from build123d import *

# Parameters (mm, degrees)
P_IDAT_VYSUNUT_M1_DEPTH  = 20
P_IDAT_VYSUNUT_M2_DEPTH  = 10
P_IDAT_START             = -16
P_IDAT_VYSUNUT_M3_DEPTH  = 12
ODEBRAT_START            = -4
SKICA4_R                 = 4.1
ODEBRAT_VYSUNUT_M1_DEPTH = 56.078274453
ODEBRAT_VYSUNUT_M5_REACH = 59.987
SKICA11_R                = 2.1
ODEBRAT_VYSUNUT_M6_REACH = 58.573
SKICA12_R                = 2.8
ZKOSEN_2_SIZE            = 2
P_IDAT_START_2           = 1
SKICA13_R                = 4.5
SKICA13_R_2              = 2.8
P_IDAT_VYSUNUT_M5_DEPTH  = 1


with BuildPart() as part:
    # Skica1 → Přidat vysunutím1 (new body)
    with BuildSketch(Plane.XY):
        Polygon((-14.43375673, 3), (-16.165807537, 0), (-8.082903769, -14), (8.082903769, -14), (16.165807537, 0), (14.43375673, 3), (16.743157806, 3), (18.475208614, 0), (9.237604307, -16), (-9.237604307, -16), (-18.475208614, 0), (-16.743157806, 3), align=None)
    extrude(amount=P_IDAT_VYSUNUT_M1_DEPTH)

    # Skica2 → Přidat vysunutím2 (add)
    with BuildSketch(Plane.XY.offset(10)):
        Polygon((-9.237604307, -16), (-29.237604307, -16), (-29.237604307, -4), (-16.165807537, -4), align=None)
    extrude(amount=P_IDAT_VYSUNUT_M2_DEPTH)

    # Skica3 → Přidat vysunutím3 (add)
    with BuildSketch(Plane(origin=(0, 0, 0), x_dir=(1, 0, 0), z_dir=(0, 1, 0)).offset(P_IDAT_START)):
        with BuildLine():
            Line((-29.237604307, -12.1), (-29.237604307, -10))
            Line((-29.237604307, -10), (-26.913048987, -10))
            ThreePointArc((-26.913048987, -10), (-32.955273849, -6.005695924), (-39.299782134, -9.5))
            Line((-39.299782134, -9.5), (-53.237604307, -9.5))
            Line((-53.237604307, -9.5), (-53.237604307, -12))
            Line((-53.237604307, -12), (-37.213783377, -12))
            ThreePointArc((-37.213783377, -12), (-33.186205288, -8.900322191), (-29.237604307, -12.1))
        make_face()
        with BuildLine():
            Line((-53.237604307, -14), (-53.237604307, -16.5))
            Line((-53.237604307, -16.5), (-39.299782134, -16.5))
            ThreePointArc((-39.299782134, -16.5), (-36.737604307, -19.062177826), (-33.237604307, -20))
            Line((-33.237604307, -20), (-29.237604307, -20))
            Line((-29.237604307, -20), (-29.237604307, -13.9))
            ThreePointArc((-29.237604307, -13.9), (-33.186205288, -17.099677809), (-37.213783377, -14))
            Line((-37.213783377, -14), (-53.237604307, -14))
        make_face()
    extrude(amount=P_IDAT_VYSUNUT_M3_DEPTH)

    # Skica4 → Odebrat vysunutím1 (cut, through all)
    with BuildSketch(Plane(origin=(0, 0, 0), x_dir=(1, 0, 0), z_dir=(0, 1, 0)).offset(ODEBRAT_START)):
        with Locations((-33.237604307, -13)):
            Circle(SKICA4_R)
    extrude(amount=-ODEBRAT_VYSUNUT_M1_DEPTH, mode=Mode.SUBTRACT)

    # Skica11 → Odebrat vysunutím5 (cut, up to next)
    with BuildSketch(Plane.XY.offset(16.5), mode=Mode.PRIVATE) as odebrat_vysunut_m5_sk1:
        with Locations((-47.237604307, -10)):
            Circle(SKICA11_R)
    odebrat_vysunut_m5_tool1 = extrude(odebrat_vysunut_m5_sk1.sketch, amount=-ODEBRAT_VYSUNUT_M5_REACH, mode=Mode.PRIVATE) & part.part
    add(odebrat_vysunut_m5_tool1.solids().sort_by_distance((-47.237604, -10, 16.5))[0], mode=Mode.SUBTRACT)

    # Skica12 → Odebrat vysunutím6 (cut, up to next)
    with BuildSketch(Plane(origin=(0, 0, 9.5), x_dir=(-1, 0, 0), z_dir=(0, 0, -1)), mode=Mode.PRIVATE) as odebrat_vysunut_m6_sk1:
        with Locations((47.237604307, -10)):
            Circle(SKICA12_R)
    odebrat_vysunut_m6_tool1 = extrude(odebrat_vysunut_m6_sk1.sketch, amount=-ODEBRAT_VYSUNUT_M6_REACH, mode=Mode.PRIVATE) & part.part
    add(odebrat_vysunut_m6_tool1.solids().sort_by_distance((-47.237604, -10, 9.5))[0], mode=Mode.SUBTRACT)

    # Zkosení2
    zkosen_2_edges = [part.edges().sort_by_distance(p)[0] for p in [
        (-53.237604307, -4, 10.75),
        (-53.237604307, -16, 10.75),
        (-53.237604307, -4, 15.25),
        (-53.237604307, -16, 15.25),
    ]]
    chamfer(zkosen_2_edges, length=ZKOSEN_2_SIZE)

    # Skica13 → Přidat vysunutím5 (add)
    with BuildSketch(Plane(origin=(0, 0, 9.5), x_dir=(-1, 0, 0), z_dir=(0, 0, -1)).offset(P_IDAT_START_2)):
        with Locations((47.237604307, -10)):
            Circle(SKICA13_R)
        with Locations((47.237604307, -10)):
            Circle(SKICA13_R_2, mode=Mode.SUBTRACT)
    extrude(amount=-P_IDAT_VYSUNUT_M5_DEPTH)


solid = part.part
Part model, mm, in its own coordinate system. A direction names the side the tool comes from. Coordinates: 2 decimals unless noted, no trailing zeros. Write each loop counter-clockwise with the first axis right and the second up, starting at its lowest first coordinate (ties: lowest second). Pieces come first, ordered by that corner, then holes. Notation, with made-up numbers: M 57.25,62.5 L 62.25,62.5 A22 cw 62.25,90.5 Z; hole C -9.5,83 d4. An arc over 180 degrees is marked long. Return JSON: item names as keys, results as strings.
1. 3-axis set-ups, long thin cutter, end or side, ignore diameter. For faces 4 (the face through (-14.82, -6.33, 7.64)), 5 (the face through (12.068, -7.098, 9.86)), 6 (the face through (-52.25, -5.01, 10.73)), 7 (the face through (-43, -10, 14)), 8 (the face through (-44.8, -10.1, 16.5)): which of +Z, -Z, +X, -X, +Y, -Y reach the whole face in a straight line?
Determined:
{"face 4": "-Z", "face 5": "+Z, -Z", "face 6": "+Z, -Z, -X, +Y", "face 7": "-X, +Y, -Y", "face 8": "+Z, -X, +Y, -Y"}
2. Saw through at A-A, the plane y = -10. Count the separate pieces of the cut face and the enclosed holes in it, then the cut area to 3 significant figures.
Determined:
{"separate pieces": "4", "enclosed holes": "0", "area": "380 mm²"}
3. Flat gauge pins, fed straight in: pin 1 Ø10 at (x, y) = (-38.5, -11.5) entering from -Z; pin 2 Ø6.5 at (x, y) = (-47.24, -10) entering from +Z; pin 3 Ø5 at (x, z) = (0, 12) entering from +Y. Where does each tip first touch, or does it go through?
Determined:
{"pin 1": "z = 6", "pin 2": "z = 16.5", "pin 3": "y = -14"}
4. Probe L1, parallel to Z at x = -41, y = -14.75; L2, parallel to X at y = -7, z = 7.75; L3, parallel to X at y = -4.5, z = 7.75. List the from-to ranges inside material, lowest first.
Determined:
{"L1": "9.5 to 12, 14 to 16.5", "L2": "-37.87 to -28.61, -14.43 to -12.12, 12.12 to 14.43", "L3": "-37.87 to -28.61, -15.88 to -13.57, 13.57 to 15.88"}
5. Saw through at B-B, the plane x = -30. Write the cut outline in (y, z).
Determined:
{"outline": "M -16,6.79 L -4,6.79 L -4,10.48 L -16,10.48 Z; M -16,15.52 L -4,15.52 L -4,20 L -16,20 Z"}
6. Saw through at D-D, the plane x = -43.5. Write the cut outline in (y, z).
Determined:
{"outline": "M -16,9.5 L -12.51,9.5 L -12.51,8.5 L -7.49,8.5 L -7.49,9.5 L -4,9.5 L -4,12 L -16,12 Z; M -16,14 L -4,14 L -4,16.5 L -16,16.5 Z"}
7. Pull direction Y, two halves, no side cores. Call faces 1 (the face through (15.3, 1.5, 9.9)), 2 (the face through (-52.25, -14.99, 15.23)), 3 (the face through (-53.238, -10, 11)): pulls with the +Y half, pulls with the -Y half, needs draft (parallel to the pull), parting line crosses it, or undercut.
Determined:
{"face 1": "undercut", "face 2": "pulls with the -Y half", "face 3": "needs draft"}
8. Saw through at C-C, the plane z = 5. Write the cut outline in (x, y), then the cut area to 3 significant figures.
Determined:
{"outline": "M -18.48,0 L -9.24,-16 L 9.24,-16 L 18.48,0 L 16.74,3 L 14.43,3 L 16.17,0 L 8.08,-14 L -8.08,-14 L -16.17,0 L -14.43,3 L -16.74,3 Z", "area": "118 mm²"}
